from build123d import *

# Parameters (mm, degrees)
REVOLVE_1_OUTLINE_W   = 0.355269541
REVOLVE_1_OUTLINE_H   = 0.438478825
REVOLVE_1_OUTLINE_W_2 = 11.364624133
REVOLVE_1_OUTLINE_W_3 = 4.372569082
REVOLVE_1_OUTLINE_H_2 = 55.75634902
REVOLVE_1_OUTLINE_H_3 = 1.854936884
REVOLVE_1_OUTLINE_W_4 = 14.211965544
REVOLVE_1_OUTLINE_H_4 = 0.61022171
SKETCH_2_R            = 30
EXTRUDE_1_DEPTH       = 30
SKETCH_3_R            = 7.5
EXTRUDE_2_DEPTH       = 37.14
SKETCH_4_W            = 5
SKETCH_4_H            = 22.5
SKETCH_4_W_2          = 22.5
SKETCH_4_H_2          = 5
EXTRUDE_3_DEPTH       = 2


# Read off the part's stored shape, not the designer's step: 회전1
with BuildPart() as part:
    # 회전1 outline → 회전1 (revolve)
    with BuildSketch(Plane.YX):
        with Locations((41.542258903, -28.097413923)):
            Rectangle(REVOLVE_1_OUTLINE_W, REVOLVE_1_OUTLINE_H)
        with BuildLine():
            add(Edge.make_bspline(
                [(41.719893674, -27.87817451), (41.894749248, -27.921618592), (42.252720208, -28.01137838), (42.873298399, -28.15700866), (43.341279515, -28.256769587), (43.642191366, -28.316653335)],
                knots=[0.117139278, 0.117139278, 0.117139278, 0.117139278, 0.14529069, 0.173442101, 0.224513922, 0.224513922, 0.224513922, 0.224513922], degree=3))
            Line((41.719893674, -27.87817451), (41.719893674, -28.316653335))
            Line((41.719893674, -28.316653335), (43.642191366, -28.316653335))
        make_face()
        with BuildLine():
            add(Edge.make_bspline(
                [(43.642191366, -28.316653335), (43.673012094, -28.322786894), (44.367114713, -28.459908676), (46.367881136, -28.788520691), (49.637320271, -29.015805628), (53.021708434, -28.821695589), (55.131271584, -28.478533008), (55.931859218, -28.316653335)],
                knots=[0.224513922, 0.224513922, 0.224513922, 0.224513922, 0.229744924, 0.34235057, 0.567561862, 0.792773154, 0.932194296, 0.932194296, 0.932194296, 0.932194296], degree=3))
            Line((43.642191366, -28.316653335), (41.719893674, -28.316653335))
            Line((41.719893674, -28.316653335), (41.719893674, -30.171590219))
            Line((41.719893674, -30.171590219), (55.931859218, -30.171590219))
            Line((55.931859218, -30.171590219), (55.931859218, -28.316653335))
        make_face()
        with Locations((35.682312067, -28.097413923)):
            Rectangle(REVOLVE_1_OUTLINE_W_2, REVOLVE_1_OUTLINE_H)
        with Locations((58.118143759, -28.097413923)):
            Rectangle(REVOLVE_1_OUTLINE_W_3, REVOLVE_1_OUTLINE_H)
        with Locations((58.118143759, 0)):
            Rectangle(REVOLVE_1_OUTLINE_W_3, REVOLVE_1_OUTLINE_H_2)
        with BuildLine():
            Line((41.719893674, 28.316653335), (41.719893674, 27.87817451))
            add(Edge.make_bspline(
                [(43.128876316, 28.316653335), (42.973861456, 28.272694047), (42.669494175, 28.183372992), (42.227403007, 28.044794313), (41.884836208, 27.931979132), (41.719893674, 27.87817451)],
                knots=[0.937972384, 0.937972384, 0.937972384, 0.937972384, 0.966974102, 0.995182728, 1.023391355, 1.023391355, 1.023391355, 1.023391355], degree=3))
            Line((43.128876316, 28.316653335), (41.719893674, 28.316653335))
        make_face()
        with Locations((41.542258903, 28.097413923)):
            Rectangle(REVOLVE_1_OUTLINE_W, REVOLVE_1_OUTLINE_H)
        with Locations((41.542258903, -29.244121777)):
            Rectangle(REVOLVE_1_OUTLINE_W, REVOLVE_1_OUTLINE_H_3)
        with Locations((58.118143759, -29.244121777)):
            Rectangle(REVOLVE_1_OUTLINE_W_3, REVOLVE_1_OUTLINE_H_3)
        with Locations((35.682312067, -29.244121777)):
            Rectangle(REVOLVE_1_OUTLINE_W_2, REVOLVE_1_OUTLINE_H_3)
        with Locations((35.682312067, 28.097413923)):
            Rectangle(REVOLVE_1_OUTLINE_W_2, REVOLVE_1_OUTLINE_H)
        with Locations((58.118143759, 28.097413923)):
            Rectangle(REVOLVE_1_OUTLINE_W_3, REVOLVE_1_OUTLINE_H)
        with BuildLine():
            Line((41.719893674, 28.316653335), (43.128876316, 28.316653335))
            add(Edge.make_bspline(
                [(55.931859218, 28.316653335), (55.350466054, 28.484554725), (54.483083768, 28.700477141), (53.332821917, 28.919070087), (52.621816991, 29.026887301), (51.140275095, 29.207221888), (48.779721438, 29.304602769), (45.95584246, 28.998713875), (44.028351242, 28.564756145), (43.275412999, 28.358208372), (43.128876316, 28.316653335)],
                knots=[0.120715306, 0.120715306, 0.120715306, 0.120715306, 0.233549812, 0.285972839, 0.342390092, 0.370598718, 0.57205333, 0.797722342, 0.910556849, 0.937972384, 0.937972384, 0.937972384, 0.937972384], degree=3))
            Line((55.931859218, 28.316653335), (55.931859218, 30.171590219))
            Line((55.931859218, 30.171590219), (41.719893674, 30.171590219))
            Line((41.719893674, 30.171590219), (41.719893674, 28.316653335))
        make_face()
        with Locations((41.542258903, 29.244121777)):
            Rectangle(REVOLVE_1_OUTLINE_W, REVOLVE_1_OUTLINE_H_3)
        with Locations((48.825876446, -30.476701074)):
            Rectangle(REVOLVE_1_OUTLINE_W_4, REVOLVE_1_OUTLINE_H_4)
        with Locations((41.542258903, -30.476701074)):
            Rectangle(REVOLVE_1_OUTLINE_W, REVOLVE_1_OUTLINE_H_4)
        with BuildLine():
            Line((60.3044283, -30.171590219), (55.931859218, -30.171590219))
            Line((55.931859218, -30.171590219), (55.931859218, -30.781811929))
            Line((55.931859218, -30.781811929), (58.176696805, -30.781811929))
            add(Edge.make_bspline(
                [(60.3044283, -30.171590219), (59.242057092, -30.511353598), (58.176696805, -30.781811929)],
                knots=[0, 0, 0, 0.113573553, 0.113573553, 0.113573553], degree=2))
        make_face()
        with Locations((35.682312067, -30.476701074)):
            Rectangle(REVOLVE_1_OUTLINE_W_2, REVOLVE_1_OUTLINE_H_4)
        with Locations((35.682312067, 29.244121777)):
            Rectangle(REVOLVE_1_OUTLINE_W_2, REVOLVE_1_OUTLINE_H_3)
        with Locations((58.118143759, 29.244121777)):
            Rectangle(REVOLVE_1_OUTLINE_W_3, REVOLVE_1_OUTLINE_H_3)
        with Locations((41.542258903, 30.476701074)):
            Rectangle(REVOLVE_1_OUTLINE_W, REVOLVE_1_OUTLINE_H_4)
        with Locations((48.825876446, 30.476701074)):
            Rectangle(REVOLVE_1_OUTLINE_W_4, REVOLVE_1_OUTLINE_H_4)
        with BuildLine():
            Line((55.931859218, -30.781811929), (41.719893674, -30.781811929))
            Line((41.719893674, -30.781811929), (41.719893674, -30.868243844))
            add(Edge.make_bspline(
                [(49.816181075, -31.837257545), (45.788933817, -31.837257541), (41.719893674, -30.868243844)],
                knots=[0.556786778, 0.556786778, 0.556786778, 0.981464752, 0.981464752, 0.981464752], degree=2))
            add(Edge.make_bspline(
                [(55.931859218, -31.274158213), (52.886163188, -31.837257547), (49.816181075, -31.837257545)],
                knots=[0.233053543, 0.233053543, 0.233053543, 0.556786778, 0.556786778, 0.556786778], degree=2))
            Line((55.931859218, -31.274158213), (55.931859218, -30.781811929))
        make_face()
        with BuildLine():
            Line((41.719893674, -30.868243844), (41.719893674, -30.781811929))
            Line((41.719893674, -30.781811929), (41.364624133, -30.781811929))
            add(Edge.make_bspline(
                [(41.719893674, -30.868243844), (41.54229871, -30.825950834), (41.364624133, -30.781811929)],
                knots=[0.981464752, 0.981464752, 0.981464752, 1, 1, 1], degree=2))
        make_face()
        with BuildLine():
            Line((58.176696805, -30.781811929), (55.931859218, -30.781811929))
            Line((55.931859218, -30.781811929), (55.931859218, -31.274158213))
            add(Edge.make_bspline(
                [(58.176696805, -30.781811929), (57.055932041, -31.066335551), (55.931859218, -31.274158213)],
                knots=[0.113573553, 0.113573553, 0.113573553, 0.233053543, 0.233053543, 0.233053543], degree=2))
        make_face()
        with Locations((35.682312067, 30.476701074)):
            Rectangle(REVOLVE_1_OUTLINE_W_2, REVOLVE_1_OUTLINE_H_4)
        with BuildLine():
            Line((55.931859218, 30.781811929), (55.931859218, 30.171590219))
            Line((55.931859218, 30.171590219), (60.3044283, 30.171590219))
            add(Edge.make_bspline(
                [(58.176696805, 30.781811929), (59.242057092, 30.511353598), (60.3044283, 30.171590219)],
                knots=[0.886426447, 0.886426447, 0.886426447, 1, 1, 1], degree=2))
            Line((58.176696805, 30.781811929), (55.931859218, 30.781811929))
        make_face()
        with BuildLine():
            Line((41.364624133, 30.781811929), (41.719893674, 30.781811929))
            Line((41.719893674, 30.781811929), (41.719893674, 30.868243844))
            add(Edge.make_bspline(
                [(41.364624133, 30.781811929), (41.54229871, 30.825950834), (41.719893674, 30.868243844)],
                knots=[0, 0, 0, 0.018535248, 0.018535248, 0.018535248], degree=2))
        make_face()
        with BuildLine():
            Line((41.719893674, 30.868243844), (41.719893674, 30.781811929))
            Line((41.719893674, 30.781811929), (55.931859218, 30.781811929))
            Line((55.931859218, 30.781811929), (55.931859218, 31.274158213))
            add(Edge.make_bspline(
                [(49.816181262, 31.837257545), (52.886163281, 31.83725753), (55.931859218, 31.274158213)],
                knots=[0.443213232, 0.443213232, 0.443213232, 0.766946457, 0.766946457, 0.766946457], degree=2))
            add(Edge.make_bspline(
                [(41.719893674, 30.868243844), (45.788933912, 31.837257564), (49.816181262, 31.837257545)],
                knots=[0.018535248, 0.018535248, 0.018535248, 0.443213232, 0.443213232, 0.443213232], degree=2))
        make_face()
        with BuildLine():
            Line((55.931859218, 31.274158213), (55.931859218, 30.781811929))
            Line((55.931859218, 30.781811929), (58.176696805, 30.781811929))
            add(Edge.make_bspline(
                [(55.931859218, 31.274158213), (57.055932041, 31.066335551), (58.176696805, 30.781811929)],
                knots=[0.766946457, 0.766946457, 0.766946457, 0.886426447, 0.886426447, 0.886426447], degree=2))
        make_face()
    revolve(axis=Axis((0, 0, 0), (1, 0, 0)))

    # 스케치2 → 보스-돌출1 (add, symmetric)
    with BuildSketch(Plane(origin=(0, 0, 0), x_dir=(0, 0, -1), z_dir=(1, 0, 0))):
        with Locations(Location((0, 0, 0), (0, 0, 270))):
            Circle(SKETCH_2_R)
    extrude(amount=EXTRUDE_1_DEPTH, both=True)

    # 스케치3 → 보스-돌출2 (add)
    with BuildSketch(Plane.ZY.offset(30)):
        with Locations(Location((0, 0, 0), (0, 0, 180))):
            Circle(SKETCH_3_R)
    extrude(amount=EXTRUDE_2_DEPTH)

    # 스케치4 → 보스-돌출3 (add)
    with BuildSketch(Plane(origin=(30, 0, 0), x_dir=(0, 0, -1), z_dir=(1, 0, 0))):
        with Locations((0, 13.75)):
            Rectangle(SKETCH_4_W, SKETCH_4_H)
        with Locations((-13.75, 0)):
            Rectangle(SKETCH_4_W_2, SKETCH_4_H_2)
        Rectangle(SKETCH_4_W, SKETCH_4_H_2)
        with Locations((13.75, 0)):
            Rectangle(SKETCH_4_W_2, SKETCH_4_H_2)
        with Locations((0, -13.75)):
            Rectangle(SKETCH_4_W, SKETCH_4_H)
    extrude(amount=EXTRUDE_3_DEPTH)


solid = part.part
Source: CAD feature listing. Evaluate the final solid. Frame: model axes, mm. A direction names the side the tool comes from. Give positions to 0.01 mm unless a question says otherwise; leave off trailing zeros. Write each loop counter-clockwise with the first axis right and the second up, starting at its lowest first coordinate (ties: lowest second). Pieces come first, ordered by that corner, then holes. Notation, with made-up numbers: (10, -9.5) - (38, -9.5) arc R16 ccw to (38, -3.5) - close; hole circle Ø3 at (-21, 33). An arc over 180 degrees is marked (long way). Write item = value, one per line. Start each with the question number.
Q1. Draft query along X for faces 5 (the flat face through (-30.782, -21, 22)), 6 (the flat face through (27.878, -18, -27)), 7 (the cylindrical face through (-30.396, 27.712, -11.49)). Return one class per face: +X half, -X half, draft (parallel to the pull), parting line (faces both ways), or undercut.
Q2. Reachability of faces 1 (the cylindrical face through (0.42, -13.07, -58.87)), 2 (the cylindrical face through (-0.396, 51.667, -21.422)), 3 (the flat face through (-30, -6, 6)), 4 (the cylindrical face through (30.385, 27.712, -11.49)) from +Z, -Z, +X, -X, +Y, -Y: full face, straight path, thin tool, end or side. Return the list, or none.
Q3. Cut plane A-A, the plane x = -23.5. Return loops of the section in (y, z), then the cut area to 3 significant figures.
Q4. Pin query (flat end, axial travel): pin 1 Ø1 at (x, z) = (30.5, -15.5) entering from +Y; pin 2 Ø6 at (x, y) = (-16, -48) entering from -Z; pin 3 Ø4 at (x, y) = (-6, 36.5) entering from +Z; pin 4 Ø10 at (x, z) = (-40, -39) entering from +Y. Return the tip coordinate at first contact, or that it passes through.
Q5. Material intervals for probe 1 along X at (y, z) = (43, 25); probe 2 along Z at (x, y) = (7, 0); probe 3 along Z at (x, y) = (3, -2), sorted ascending.
Q6. Cut plane B-B, the plane y = 0. Give the number of separate pieces and of enclosed holes in the cut face, then the cut area to 3 significant figures.
Computed values:
q1.face_5 = -X half
q1.face_6 = undercut
q1.face_7 = draft
q2.face_1 = +X, -X
q2.face_2 = none
q2.face_3 = -X
q2.face_4 = +X
q3.outline = circle Ø120.61 at (0, 0); circle Ø60 at (0, 0); hole circle Ø111.86 at (0, 0)
q3.area = 4,420 mm²
q4.pin_1 = 58.38
q4.pin_2 = -40.15
q4.pin_3 = 49.46
q4.pin_4 = through
q5.probe_1 = -31.84 to -28.93, 29.23 to 31.84
q5.probe_2 = -60.3 to -55.93, -30 to 30, 55.93 to 60.3
q5.probe_3 = -60.27 to -55.9, -29.93 to 29.93, 55.9 to 60.27
q6.separate_pieces = 1
q6.enclosed_holes = 2
q6.area = 5,090 mm²
